Part print with two shaded views. Sizes in mm from the minimum x, y, z corner. Round coordinates to 2 decimals unless told otherwise and drop trailing zeros. Write each loop counter-clockwise with the first axis right and the second up, starting at its lowest first coordinate (ties: lowest second). Pieces come first, ordered by that corner, then holes. Notation, with made-up numbers: (14, 11.25) - (67, 11.25) arc R26 cw to (67, 28.25) - close; hole circle Ø7 at (31.25, 49.5). An arc over 180 degrees is marked (long way). Answer as a JSON object with one key per item and string values. Group by question number.
Item 1: Flat gauge pins, fed straight in: pin 1 (3 mm diameter, centred on y = 11.5, z = 4, fed in from -X); pin 2 (6 mm diameter, centred on x = 262, z = 6.5, fed in from -Y). Where does each tip first touch, or does it go through?
Item 2: Probe line 1 (X direction, y = 3.25, z = 4.75); line 2 (Y direction, x = 74, z = 8.75) (1 decimal); line 3 (Z direction, x = 65, y = 7.5) (1 decimal). List the from-to ranges inside material, lowest first. Write a range as from..to.
Item 3: Slice it at A-A, the plane x = 237. List the corners of the cut face in (y, z).
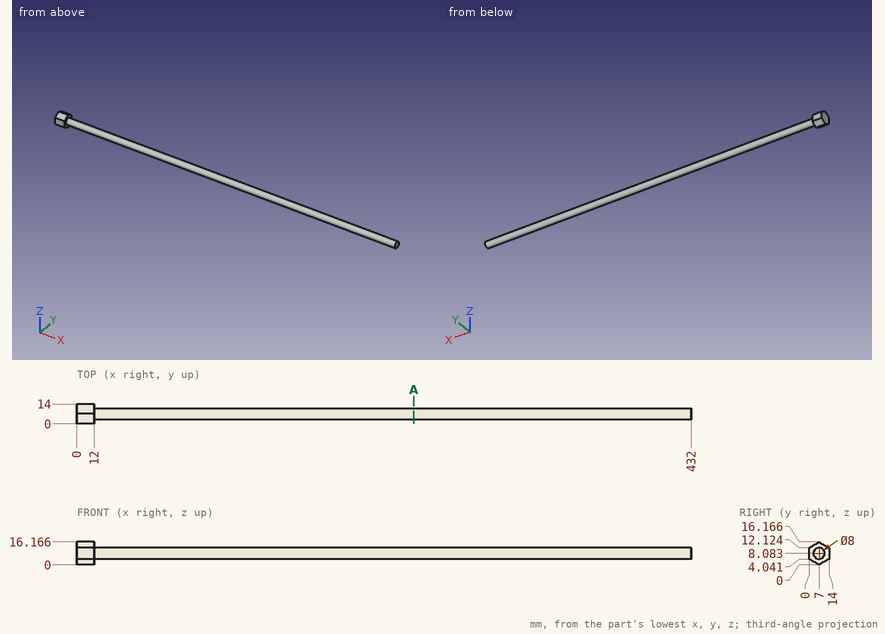
Geometry says:
{
 "1": {"pin 1": "stops at x = 0", "pin 2": "stops at y = 3"},
 "2": {"line 1": "x = 0..12", "line 2": "y = 3.1..10.9", "line 3": "z = 4.1..12.1"},
 "3": {"outline": "circle Ø8 at (7, 8.08)"}
}
